Work out the finished part from the listing and answer in its coordinate system (mm). A direction names the side the tool comes from. Round coordinates to 2 decimals unless told otherwise and drop trailing zeros. Order: outer loops, then holes, each group sorted by start corner. A loop starts at its lowest first (then second) coordinate and runs counter-clockwise, first axis right, second up. Notation, with made-up numbers: (87.5, 68) - (142.5, 68) arc R23 ccw to (142.5, 78) - close; hole circle Ø4 at (86, 22.5). An arc over 180 degrees is marked (long way). One line per question, with ' | ' between items. Start each with the question number.
from build123d import *

# Parameters (mm, degrees)
EXTRUDE_THIN1_DEPTH = 220
BOSS_EXTRUDE1_DEPTH = 10
BOSS_EXTRUDE2_DEPTH = 10
CUT_EXTRUDE1_DEPTH  = 221
SKETCH6_R           = 2.5
CUT_EXTRUDE3_DEPTH  = 221
BOSS_EXTRUDE3_DEPTH = 220
SKETCH9_W           = 89.464875501
SKETCH9_H           = 210
CUT_EXTRUDE5_DEPTH  = 25
SKETCH10_W          = 38.507874252
SKETCH10_H          = 15.616205768
CUT_EXTRUDE6_DEPTH  = 20


with BuildPart() as part:
    # Sketch1 → Extrude-Thin1 (new body)
    with BuildSketch(Plane.XY):
        with BuildLine():
            Line((-111.804811095, -25.936023273), (-1.752290831, -25.936023273))
            ThreePointArc((-1.752290831, -25.936023273), (3.519458689, -24.716035193), (7.71929628, -21.304132772))
            Line((7.71929628, -21.304132772), (21.420171512, -3.691876429))
            Line((21.420171512, -3.691876429), (8.721276915, 5.936816741))
            ThreePointArc((8.721276915, 5.936816741), (3.01180177, 8.957008398), (-3.362508592, 10))
            Line((-3.362508592, 10), (-109.847422235, 10))
            ThreePointArc((-109.847422235, 10), (-115.643105208, 9.14184053), (-120.941426159, 6.641005887))
            Line((-120.941426159, 6.641005887), (-134.097771182, -2.129890795))
            Line((-134.097771182, -2.129890795), (-121.789414627, -20.592425628))
            ThreePointArc((-121.789414627, -20.592425628), (-117.467106201, -24.516118458), (-111.804811095, -25.936023273))
        make_face()
        with BuildLine():
            Line((-111.804811095, -15.936023273), (-1.752290831, -15.936023273))
            ThreePointArc((-1.752290831, -15.936023273), (-0.873665911, -15.732691927), (-0.17369298, -15.164041523))
            Line((-0.17369298, -15.164041523), (7.310590323, -5.543114841))
            Line((7.310590323, -5.543114841), (2.679384161, -2.03159163))
            ThreePointArc((2.679384161, -2.03159163), (-0.175353411, -0.521495801), (-3.362508592, 0))
            Line((-3.362508592, 0), (-109.847422235, 0))
            ThreePointArc((-109.847422235, 0), (-112.745263722, -0.429079735), (-115.394424197, -1.679497057))
            Line((-115.394424197, -1.679497057), (-120.230266277, -4.903391776))
            Line((-120.230266277, -4.903391776), (-113.468911684, -15.045423666))
            ThreePointArc((-113.468911684, -15.045423666), (-112.748526946, -15.699372471), (-111.804811095, -15.936023273))
        make_face(mode=Mode.SUBTRACT)
    extrude(amount=EXTRUDE_THIN1_DEPTH)

    # Sketch3 → Boss-Extrude1 (add)
    with BuildSketch(Plane.XY.offset(220)):
        Polygon((-120.230266277, -4.903391776), (7.310590323, -5.543114841), (7.310590323, -21.801402169), (-120.525433927, -22.179247), align=None)
    extrude(amount=-BOSS_EXTRUDE1_DEPTH)

    # Sketch4 → Boss-Extrude2 (add)
    with BuildSketch(Plane(origin=(0, 0, 0), x_dir=(-1, 0, 0), z_dir=(0, 0, -1))):
        Polygon((-7.310590323, -5.543114841), (120.230266277, -4.903391776), (120.230266277, -22.480711973), (-5.288915881, -22.480711973), (-7.235397459, -20.534230396), align=None)
    extrude(amount=-BOSS_EXTRUDE2_DEPTH)

    # Sketch5 → Cut-Extrude1 (cut, through all)
    with BuildSketch(Plane(origin=(0, 0, 0), x_dir=(-1, 0, 0), z_dir=(0, 0, -1))):
        Polygon((-7.310590323, -5.543114841), (-30.090389748, -5.543114841), (-30.090389748, 22.160064079), (140.461111039, 22.160064079), (140.461111039, -4.844552144), (120.230266277, -4.903391776), align=None)
    extrude(amount=-CUT_EXTRUDE1_DEPTH, mode=Mode.SUBTRACT)

    # Sketch6 → Cut-Extrude3 (cut, through all)
    with BuildSketch(Plane.XY.offset(220)):
        with Locations((-106.752290831, -11.972659606)):
            Circle(SKETCH6_R)
        with Locations((-6.752290831, -11.972659606)):
            Circle(SKETCH6_R)
        with Locations((-86.752290831, -11.972659606)):
            Circle(SKETCH6_R)
        with Locations((-66.752290831, -11.972659606)):
            Circle(SKETCH6_R)
        with Locations((-46.752290831, -11.972659606)):
            Circle(SKETCH6_R)
        with Locations((-26.752290831, -11.972659606)):
            Circle(SKETCH6_R)
    extrude(amount=-CUT_EXTRUDE3_DEPTH, mode=Mode.SUBTRACT)

    # Sketch8 → Boss-Extrude3 (add)
    with BuildSketch(Plane.XY.offset(220)):
        with BuildLine():
            Line((-107.467244942, 17.002107807), (-6.002369441, 17.002107807))
            ThreePointArc((-6.002369441, 17.002107807), (-2.090901759, 16.205390949), (1.197299473, 13.942191923))
            Line((1.197299473, 13.942191923), (19.98006151, -5.543114841))
            Line((19.98006151, -5.543114841), (7.310590323, -5.543114841))
            Line((7.310590323, -5.543114841), (-120.230266277, -4.903391776))
            Line((-120.230266277, -4.903391776), (-132.272118974, -4.868369107))
            Line((-132.272118974, -4.868369107), (-114.768654919, 13.835072929))
            ThreePointArc((-114.768654919, 13.835072929), (-111.446588404, 16.176246765), (-107.467244942, 17.002107807))
        make_face()
    extrude(amount=-BOSS_EXTRUDE3_DEPTH)

    # Sketch9 → Cut-Extrude5 (cut)
    with BuildSketch(Plane(origin=(0, 17.002107807, 0), x_dir=(1, 0, 0), z_dir=(0, 1, 0))):
        with Locations((-50.734807192, -110)):
            Rectangle(SKETCH9_W, SKETCH9_H)
    extrude(amount=-CUT_EXTRUDE5_DEPTH, mode=Mode.SUBTRACT)

    # Sketch10 → Cut-Extrude6 (cut)
    with BuildSketch(Plane(origin=(-68.086200957, 63.717917206, 0), x_dir=(0, 0, 1), z_dir=(-0.730140998, 0.683296512, 0))):
        with Locations((110, -82.127570542)):
            Rectangle(SKETCH10_W, SKETCH10_H)
    extrude(amount=-CUT_EXTRUDE6_DEPTH, mode=Mode.SUBTRACT)


solid = part.part
1) Flat-ended cylindrical pins translate along their axes: pin 1 (4 mm diameter, centred on x = -47.5, z = 212.5, fed in from +Y); pin 2 (1 mm diameter, centred on y = -15.5, z = 49, fed in from -X); pin 3 (20 mm diameter, centred on y = 4, z = 116.5, fed in from -X). Find the tip coordinate at first contact, or state that the pin passes through.
2) Determine the mould class of faces 1 (the flat face through (-58, -25.936, 108)), 2 (the flat face through (-51, -7.998, 7)), 3 (the cylindrical face through (-49.25, -11.86, 215.07)) for opening direction Y: released by +Y, released by -Y, zero draft, split by the parting line, or undercut.
3) Straight lines are drawn through the part: line 1 (Z direction, x = -51, y = -5); line 2 (Z direction, x = -109, y = -0.5); line 3 (Y direction, x = -20, z = 159). For each, find the intervals that lie inside material, in ascending order.
4) Section B-B on x = -38.5 is taken. Give the vertices of the cut face in (y, z).
5) Section C-C on z = 160 is taken. Give the vertices of the cut face in (x, y), and give its area (3 significant figures).
6) Section A-A on z = 121 is taken. Give the vertices of the cut face in (x, y).
7) Section D-D on y = 2.5 is taken. Give the vertices of the cut face in (x, z).
8) For faces 4 (the flat face through (-117.808, 10.587, 111.54)), 5 (the flat face through (-51, 5, 215)), 6 (the flat face through (-57, -12, 10)), determine the directions among +Z, -Z, +X, -X, +Y, -Y from which every point of the face is accessible in a straight line to the end or side of a thin tool.
Recorded:
1) pin 1: stops at y = -8 | pin 2: stops at x = -125.52 | pin 3: stops at x = -132.27
2) face 1: released by -Y | face 2: released by +Y | face 3: undercut
3) line 1: z = 0 to 5, 215 to 220 | line 2: z = 0 to 90.75, 129.25 to 220 | line 3: y = -25.94 to -15.94
4) outline: (-25.94, 0) - (17, 0) - (17, 5) - (-8, 5) - (-8, 10) - (-15.94, 10) - (-15.94, 210) - (-8, 210) - (-8, 215) - (17, 215) - (17, 220) - (-25.94, 220) - close
5) outline: (-132.27, -4.87) - (-121.79, -20.59) arc R12 ccw to (-111.8, -25.94) - (-1.75, -25.94) arc R12 ccw to (7.72, -21.3) - (19.98, -5.54) - (1.2, 13.94) arc R10 ccw to (-6, 17) - (-6, -5.48) - (7.31, -5.54) - (-0.17, -15.16) arc R2 cw to (-1.75, -15.94) - (-111.8, -15.94) arc R2 cw to (-113.47, -15.05) - (-120.23, -4.9) - (-95.47, -5.03) - (-95.47, 17) - (-107.47, 17) arc R10 ccw to (-114.77, 13.84) - close | area: 2,470 mm²
6) outline: (-132.27, -4.87) - (-121.79, -20.59) arc R12 ccw to (-111.8, -25.94) - (-1.75, -25.94) arc R12 ccw to (7.72, -21.3) - (19.98, -5.54) - (1.2, 13.94) arc R10 ccw to (-6, 17) - (-6, -5.48) - (7.31, -5.54) - (-0.17, -15.16) arc R2 cw to (-1.75, -15.94) - (-111.8, -15.94) arc R2 cw to (-113.47, -15.05) - (-113.86, -14.46) - (-114.94, -15.61) - (-129.54, -1.95) - close; (-118.87, 9.45) - (-104.27, -4.21) - (-104.98, -4.98) - (-95.47, -5.03) - (-95.47, 17) - (-107.47, 17) arc R10 ccw to (-114.77, 13.84) - close
7) outline: (-125.38, 0) - (12.23, 0) - (12.23, 220) - (-125.38, 220) - (-125.38, 129.25) - (-111.44, 129.25) - (-111.44, 90.75) - (-125.38, 90.75) - close; hole (-95.47, 5) - (-6, 5) - (-6, 215) - (-95.47, 215) - close
8) face 4: +Z, -Z, -X, +Y | face 5: +Y | face 6: none
